Build history of the part. All positions in model axes, mm. A direction names the side the tool comes from. Give positions to 0.01 mm unless a question says otherwise; leave off trailing zeros. Loops run counter-clockwise (first coordinate to the right, second up) from the corner with the lowest first, then second, coordinate; pieces in that order, holes last.
1) Band-saw the part on A-A on z = 21. List the corners of the cut face in (x, y).
2) Two-plate mould, pull along X, no slides. Class faces 1 (the flat face through (43, 2, -15)), 2 (the flat face through (0, 2, -22)), 3 (the flat face through (-44.5, 1, 18)), 4 (the flat face through (15, 2, 22)): +X half, -X half, draft (parallel to the pull), parting line (faces both ways), or undercut.
3) Wall check: line 1 (X direction, y = 1.5, z = 21); line 2 (Z direction, x = 39.5, y = 2); line 3 (X direction, y = 2.75, z = -6). Give the ranges that are in metal, low to high.
4) 3-axis set-ups, long thin cutter, end or side, ignore diameter. For faces 5 (the flat face through (0, 2, 20)), 6 (the flat face through (41.5, 2, 10)), 7 (the flat face through (-40, 2, -22)): which of +Z, -Z, +X, -X, +Y, -Y reach the whole face in a straight line?
5) Band-saw the part on C-C on z = -12.5. List the corners of the cut face in (x, y), then the cut area to 3 significant figures.
6) Band-saw the part on B-B on x = -1. List the corners of the cut face in (y, z).
7) Flat gauge pins, fed straight in: P1, Ø1, axis at x = 12, z = 11, coming from the -Y side; P2, Ø0.9, axis at y = 1, z = 22.5, coming from the +X side; P3, Ø0.9, axis at y = 1.5, z = 22.5, coming from the -X side; P4, Ø1.5, axis at x = 43.5, y = 1, coming from the +Z side. Where does each tip first touch, or does it go through?
Autodesk Inventor part; units mm, degrees
ref_plane "YZ Plane" through (0, 0, 0) normal (1, 0, 0) x (0, 1, 0)
ref_plane "XZ Plane" through (0, 0, 0) normal (0, 1, 0) x (-1, 0, 0)
ref_plane "XY Plane" through (0, 0, 0) normal (0, 0, 1) x (1, 0, 0)
sketch "Sketch1" plane through (0, 0, 0) normal (0, 1, 0) x (1, 0, 0)
  line L0 (44.5, -25) -> (-44.5, -25)
  line L1 (-44.5, -25) -> (-44.5, 25)
  line L2 (-44.5, 25) -> (44.5, 25)
  line L3 (44.5, 25) -> (44.5, -25)
  line L4 (44.5, -25) -> (-44.5, 25) construction
  line L5 (-44.5, -25) -> (44.5, 25) construction
  point P0 (0, 0)
  dimension "d0" = 89
  dimension "d1" = 50
extrude "Extrusion1" add sketch "Sketch1" along normal blind 3
sketch "Sketch2" plane through (0, 3, 0) normal (0, 1, 0) x (1, 0, 0)
  line L0 (44.5, 25) -> (-44.5, 25) construction
  line L1 (-5, 25) -> (5, 25)
  line L2 (5, 25) -> (5, 22)
  line L3 (5, 22) -> (-5, 22)
  line L4 (-5, 22) -> (-5, 25)
  line L5 (0, 35) -> (0, -35) construction
  point P0 (0, 0)
  dimension "d4" = 10
  dimension "d5" = 3
extrude "Extrusion2" cut sketch "Sketch2" against normal through all
pattern_linear "Rectangular Pattern1" count 3 spacing 20 along (-1, 0, 0) count 2 spacing 40 along (1, 0, 0) of "Extrusion2"
sketch "Sketch3" plane through (0, 3, 0) normal (0, 1, 0) x (1, 0, 0)
  line L0 (-44.5, -15) -> (-41.5, -15)
  line L1 (-41.5, -15) -> (-41.5, -5)
  line L2 (-41.5, -5) -> (-44.5, -5)
  line L3 (-44.5, -5) -> (-44.5, -15)
  line L4 (-44.5, 25) -> (-44.5, -25) construction
  line L5 (62.3, 0) -> (-62.3, 0) construction
  point P0 (0, 0)
  dimension "d15" = 3
  dimension "d16" = 10
  dimension "d17" = 5
extrude "Extrusion3" cut sketch "Sketch3" against normal blind 3
pattern_linear "Rectangular Pattern2" count 2 spacing 20 along (0, 0, -1) of "Extrusion3"
mirror "Mirror2" about plane through (0, 0, 0) normal (1, 0, 0) of "Extrusion3", "Rectangular Pattern2"
sketch "Sketch4" plane through (0, 3, 0) normal (0, 1, 0) x (1, 0, 0)
  line L0 (-44.5, -25) -> (44.5, -25) construction
  line L1 (-5, -25) -> (5, -25)
  line L2 (5, -25) -> (5, -20)
  line L3 (5, -20) -> (-5, -20)
  line L4 (-5, -20) -> (-5, -25)
  line L5 (0, 35) -> (0, -35) construction
  point P0 (0, 0)
  dimension "d23" = 10
  dimension "d24" = 5
extrude "Extrusion4" cut sketch "Sketch4" against normal through all
pattern_linear "Rectangular Pattern3" count 3 spacing 20 along (-1, 0, 0) count 2 spacing 40 along (1, 0, 0) of "Extrusion4"
equation "\"d0\" = Module_Height"
equation "\"d1\" = Module_Depth"
equation "\"d2\" = Module_Case_Thickness"
equation "\"d4\" = Module_Case_SlotWidth"
equation "\"d5\" = Module_Case_SlotDepth"
equation "\"d7\" = Module_Case_Thickness"
equation "\"d11\" = 2 * Module_Case_SlotWidth"
equation "\"d14\" = 4 * Module_Case_SlotWidth"
equation "\"d15\" = Module_Case_SlotDepth"
equation "\"d16\" = Module_Case_SlotWidth"
equation "\"d17\" = 0.5 * Module_Case_SlotWidth"
equation "\"d18\" = Module_Case_Thickness"
equation "\"d22\" = 2 * Module_Case_SlotWidth"
equation "\"d23\" = Module_Case_SlotWidth"
equation "\"d24\" = Module_Case_BottomSlotDepth"
equation "\"d30\" = 2 * Module_Case_SlotWidth"
equation "\"d33\" = 4 * Module_Case_SlotWidth"
equation "\"RackWidth\" = 482.6"
equation "\"U\" = 44.5"
equation "\"Module_Connector_Width\" = 6"
equation "\"Module_Case_SlotWidth\" = 10"
equation "\"Module_Case_SlotDepth\" = 3"
equation "\"Module_Depth\" = 50"
equation "\"Module_Back_Thickness\" = 5"
equation "\"Module_Connector_Depth\" = 4"
equation "\"Module_Height\" = 89"
equation "\"Module_Width\" = 96.52"
equation "\"Module_Case_Thickness\" = 3"
equation "\"Module_StatusIndicatorDiameter\" = 5"
equation "\"Module_Case_BottomSlotDepth\" = 5"
properties part number "LeftRigthPlate" material "Wood (Birch)"
Findings below:
1. outline: (-35, 0) - (-25, 0) - (-25, 3) - (-35, 3) - close; (-15, 0) - (-5, 0) - (-5, 3) - (-15, 3) - close; (5, 0) - (15, 0) - (15, 3) - (5, 3) - close; (25, 0) - (35, 0) - (35, 3) - (25, 3) - close
2. face 1: draft
2. face 2: undercut
2. face 3: -X half
2. face 4: undercut
3. line 1: x = -35 to -25, -15 to -5, 5 to 15, 25 to 35
3. line 2: z = -22 to 20
3. line 3: x = -41.5 to 41.5
4. face 5: +Z, +Y, -Y
4. face 6: +X, +Y, -Y
4. face 7: -Z, -X, +Y, -Y
5. outline: (-41.5, 0) - (41.5, 0) - (41.5, 3) - (-41.5, 3) - close
5. area: 249 mm2
6. outline: (0, -22) - (3, -22) - (3, 20) - (0, 20) - close
7. P1: stops at y = 0
7. P2: stops at x = 35
7. P3: stops at x = -35
7. P4: stops at z = 20
